from build123d import *

# Parameters (mm, degrees)
F2_R     = 15
F3_DEPTH = 10
F4_R     = 2


with BuildPart() as f1:
    # F0 (on Front) → F1 (revolve)
    with BuildSketch(Plane.XZ):
        with BuildLine():
            Line((-97.105525, 26.374421), (-97.105525, 18.469065))
            Line((-97.105525, 18.469065), (0, 18.469065))
            Line((0, 18.469065), (0, 31.374421))
            Line((0, 31.374421), (-92.105525, 31.374421))
            ThreePointArc((-92.105525, 31.374421), (-95.641059, 29.909955), (-97.105525, 26.374421))
        make_face()
    revolve(axis=Axis((0, 0, 24.921743), (0, 0, -1)))

    # F2 (on face) → F3 (join)
    with BuildSketch(Plane.XY.offset(31.374421)):
        with Locations((0.124191, -0.372573)):
            Circle(F2_R)
    extrude(amount=F3_DEPTH)

    # F4
    f4_edges = [f1.edges().sort_by_distance(p)[0] for p in [
        (-14.875809, -0.372573, 41.374421),
    ]]
    fillet(f4_edges, radius=F4_R)


solid = f1.part
Could you check a few things on this model? Use its own coordinates, in mm. A direction names the side the tool comes from. Coordinates: 2 decimals unless noted, no trailing zeros. Order: outer loops, then holes, each group sorted by start corner. A loop starts at its lowest first (then second) coordinate and runs counter-clockwise, first axis right, second up. Notation, with made-up numbers: (14.25, 74) - (56.25, 74) arc R24 ccw to (56.25, 98) - close; hole circle Ø8 at (-37.75, 37). An arc over 180 degrees is marked (long way). Answer in a Markdown table with one row per item. Add a question column.
(1) On a 3-axis mill with a long thin cutter (end or side, diameter ignored), from which of +Z, -Z, +X, -X, +Y, -Y can I reach the whole of each face in a straight line? I mean faces 1 (the face through (1, 1, 18.469)), 2 (the face through (14.432, 4.133, 35.318)). Say none if no direction works.
(2) If we section it at A-A, the plane z = 35.75: Please give me the cut outline in (x, y).
(3) Will these pins go through, and if not, where does the flat tip stop? pin 1 (3 mm diameter, centred on x = 3.5, y = -58.5, fed in from +Z); pin 2 (5 mm diameter, centred on x = 56, z = 30.5, fed in from -Y); pin 3 (12 mm diameter, centred on x = 71.5, z = 29.5, fed in from +Y).
(4) I need wall thicknesses on L1, parallel to Z at x = -24.5, y = -3.5; L2, parallel to Y at x = -8.5, z = 20.25; L3, parallel to X at y = -80, z = 23.5. Which ranges of each line are inside material? Lowest first, please.
Results are:
| question | item | result |
|---|---|---|
| 1 | face 1 | -Z, +X, -X, +Y, -Y |
| 1 | face 2 | +Z |
| 2 | outline | circle Ø30 at (0.12, -0.37) |
| 3 | pin 1 | stops at z = 31.37 |
| 3 | pin 2 | stops at y = -79.84 |
| 3 | pin 3 | stops at y = 71.2 |
| 4 | L1 | z = 18.47 to 31.37 |
| 4 | L2 | y = -96.73 to 96.73 |
| 4 | L3 | x = -55.04 to 55.04 |
